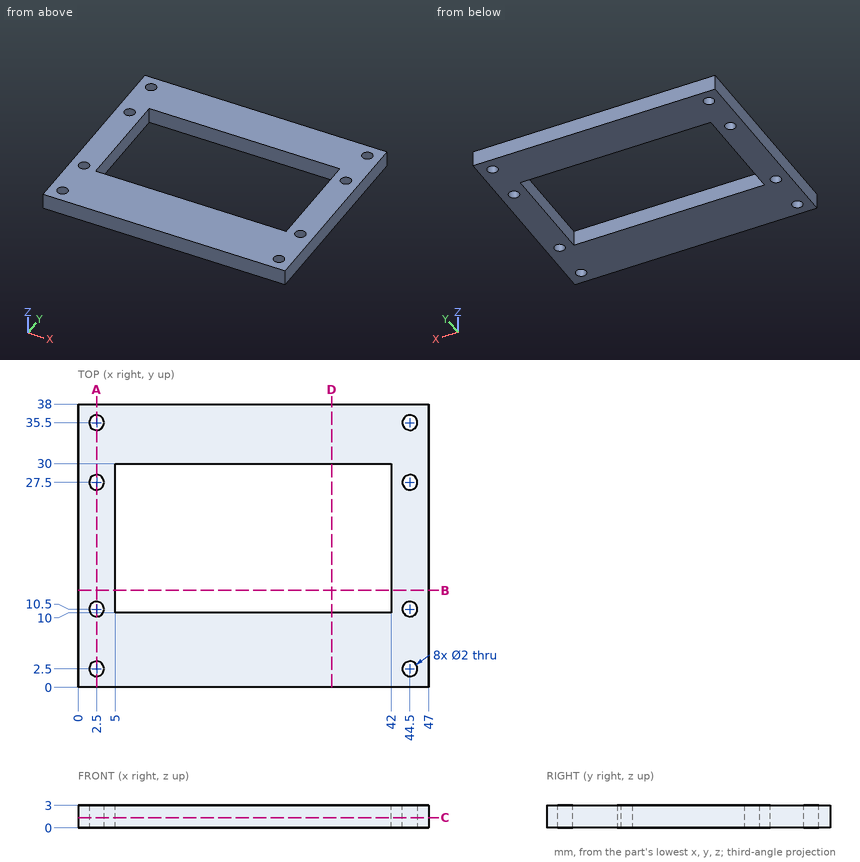
Check sheet for the drawn part. Datum: minimum x, y, z corner. Units: mm. Round coordinates to 2 decimals unless told otherwise and drop trailing zeros. Loops run counter-clockwise (first coordinate to the right, second up) from the corner with the lowest first, then second, coordinate; pieces in that order, holes last. Notation, with made-up numbers: M -36,73.5 L -3,73.5 A23 ccw -3,89.5 Z; hole C -29,-35.5 d9. An arc over 180 degrees is marked long. Write each question's results on one line, items separated by ' | '.
1) Scan lines: L1, parallel to Y at x = 44.5, z = 1.55; L2, parallel to X at y = 23.5, z = 2.55; L3, parallel to Y at x = 22, z = 2.4. Record each from-to range of solid material in increasing order. Write a range as from..to.
Checks:
L1: y = 0..1.5, 3.5..9.5, 11.5..26.5, 28.5..34.5, 36.5..38 | L2: x = 0..5, 42..47 | L3: y = 0..10, 30..38
2) Section check B-B on y = 13. Record the boundary of the cut face in (x, z), then the cut area to 3 significant figures.
Checks:
outline: M 0,0 L 5,0 L 5,3 L 0,3 Z; M 42,0 L 47,0 L 47,3 L 42,3 Z | area: 30.0 mm2
3) Gauge pin test, flat ends, axial feed: P1, Ø3, axis at x = 44.5, y = 27.5, coming from the -Z side; P2, Ø1.6, axis at x = 2.5, y = 2.5, coming from the +Z side. Record the tip position at first contact, or that the pin passes through.
Checks:
P1: stops at z = 0 | P2: passes through
4) Section check A-A on x = 2.5. Record the boundary of the cut face in (y, z).
Checks:
outline: M 0,0 L 1.5,0 L 1.5,3 L 0,3 Z; M 3.5,0 L 9.5,0 L 9.5,3 L 3.5,3 Z; M 11.5,0 L 26.5,0 L 26.5,3 L 11.5,3 Z; M 28.5,0 L 34.5,0 L 34.5,3 L 28.5,3 Z; M 36.5,0 L 38,0 L 38,3 L 36.5,3 Z
5) Section check D-D on x = 34. Record the boundary of the cut face in (y, z).
Checks:
outline: M 0,0 L 10,0 L 10,3 L 0,3 Z; M 30,0 L 38,0 L 38,3 L 30,3 Z
6) Section check C-C on z = 1.35. State how many separate pieces and enclosed holes the cut face has, then the cut area to 3 significant figures.
Checks:
separate pieces: 1 | enclosed holes: 9 | area: 1,020 mm2
